Build history of the part. All positions in model axes, mm. Coordinates: 2 decimals unless noted, no trailing zeros. Order: outer loops, then holes, each group sorted by start corner. A loop starts at its lowest first (then second) coordinate and runs counter-clockwise, first axis right, second up. Notation, with made-up numbers: (18, -18.5) - (38, -18.5) arc R35 ccw to (38, 19.5) - close; hole circle Ø11 at (12.25, -1.5). An arc over 180 degrees is marked (long way). Write each question's results on one line, items separated by ' | '.
Autodesk Inventor part; units mm, degrees
ref_plane "YZ Plane" through (0, 0, 0) normal (1, 0, 0) x (0, 1, 0)
ref_plane "XZ Plane" through (0, 0, 0) normal (0, 1, 0) x (-1, 0, 0)
ref_plane "XY Plane" through (0, 0, 0) normal (0, 0, 1) x (1, 0, 0)
sketch "Skizze1" plane through (0, 0, 0) normal (1, 0, 0) x (0, 1, 0)
  line L0 (0, -308) -> (0, 308)
  line L1 (-315, 0) -> (315, 0)
  line L2 (225, 220) -> (-225, 220)
  line L3 (-225, 220) -> (-225, -220)
  line L4 (-225, -220) -> (225, -220)
  line L5 (225, -220) -> (225, 220)
  point P0 (0, 0)
  dimension "d0" = 440
  dimension "d1" = 450
extrude "Extrusion1" add sketch "Skizze1" along normal blind 20
chamfer "Fase1" distance 20 angle 45 4 edges at (0, 0, 220) (0, 225, 0) (0, 0, -220) (0, -225, 0)
properties part number "Wand2"
1. Band-saw the part on C-C on x = 14.5. Give the cut face in (y, z).
Solved:
outline: (-219.5, -214.5) - (219.5, -214.5) - (219.5, 214.5) - (-219.5, 214.5) - close
2. Probe line 1 (Y direction, x = 10.75, z = 198); line 2 (Z direction, x = 14, y = -137); line 3 (Y direction, x = 7, z = -195). List the from-to ranges inside material, lowest first.
Solved:
line 1: y = -215.75 to 215.75 | line 2: z = -214 to 214 | line 3: y = -212 to 212
3. Drop flat-ended pins along their axis: pin 1 Ø1 at (x, z) = (5.5, 56) entering from -Y; pin 2 Ø10 at (x, y) = (9.5, -107.5) entering from -Z; pin 3 Ø6 at (x, y) = (12, -26) entering from -Z. Give the stop position or say it passes through.
Solved:
pin 1: stops at y = -211 | pin 2: stops at z = -214.5 | pin 3: stops at z = -215
